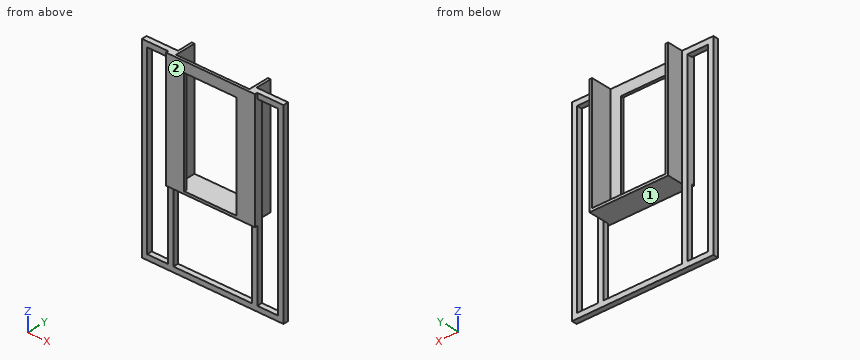
Autodesk Inventor part; units mm, degrees
ref_plane "Work Plane1" through (-336.3192, 12.7, -902.3714) normal (1, 0, 0) x (0, -1, 0)
ref_plane "YZ Plane" through (0, 0, 0) normal (1, 0, 0) x (0, 1, 0)
ref_plane "XZ Plane" through (0, 0, 0) normal (0, 1, 0) x (-1, 0, 0)
sketch "Sketch1" plane through (0, 0, 0) normal (0, 1, 0) x (-1, 0, 0)
  line L0 (-6.5808, 12.0286) -> (-6.5808, -927.7714)
  line L1 (-6.5808, 12.0286) -> (18.8192, 12.0286)
  line L2 (18.8192, 12.0286) -> (18.8192, -902.3714)
  line L3 (18.8192, -902.3714) -> (653.8192, -902.3714)
  line L4 (653.8192, -902.3714) -> (653.8192, 12.0286)
  line L5 (653.8192, 12.0286) -> (679.2192, 12.0286)
  line L6 (679.2192, 12.0286) -> (679.2192, -927.7714)
  line L7 (679.2192, -927.7714) -> (-6.5808, -927.7714)
  line L8 (18.8192, 12.0286) -> (145.8192, 12.0286)
  line L9 (145.8192, 12.0286) -> (145.8192, -902.3714)
  line L10 (145.8192, -902.3714) -> (120.4192, -902.3714)
  line L11 (120.4192, -902.3714) -> (120.4192, 12.0286)
  line L12 (120.4192, -13.8644) -> (18.8192, -13.8644)
  line L13 (653.8192, 12.0286) -> (526.8192, 12.0286)
  line L14 (526.8192, 12.0286) -> (526.8192, -902.3714)
  line L15 (552.2192, 12.0286) -> (552.2192, -902.3714)
  line L16 (552.2192, -13.8644) -> (653.8192, -13.8644)
  point P0 (69.6192, -13.8644)
  dimension "d0" = 939.8
  dimension "d1" = 25.4
  dimension "d2" = 914.4
  dimension "d3" = 635
  dimension "d5" = 25.4
  dimension "d6" = 90
  dimension "d9" = 127
  dimension "d11" = 25.4
  dimension "d12" = 127
  dimension "d21" = 25.4
extrude "Extrusion1" add sketch "Sketch1" along normal mid plane 25.4 contours L1 L2 L3 L4 L5 L6 L7 L0 | L8 L11 L12 L2 | L8 L9 L3 L11 | L4 L16 L15 L13 | L15 L3 L14 L13
sketch "Sketch2" plane through (-526.8192, -12.7, -902.3714) normal (1, 0, 0) x (0, 0, -1)
  line L0 (-914.4, 0) -> (-355.6, 0)
  line L1 (-355.6, 0) -> (-355.6, 101.6)
  line L2 (-355.6, 101.6) -> (-914.4, 101.6)
  line L3 (-914.4, 101.6) -> (-914.4, 0)
  dimension "d14" = 558.8
  dimension "d16" = 101.6
extrude "Extrusion2" add sketch "Sketch2" along normal blind 12.7
ref_plane "Work Plane1" through (-336.3192, 12.7, -902.3714) normal (1, 0, 0) x (0, -1, 0)
mirror "Mirror1" about plane through (-336.3192, 12.7, -902.3714) normal (1, 0, 0) of "Extrusion2"
sketch "Sketch3" plane through (-145.8192, 12.7, -546.7714) normal (0, 0, -1) x (-1, 0, 0)
  line L0 (0, 76.2) -> (381, 76.2)
  line L1 (381, 76.2) -> (381, -25.4)
  line L2 (381, -25.4) -> (0, -25.4)
  line L3 (0, -25.4) -> (0, 76.2)
extrude "Extrusion3" add sketch "Sketch3" along normal blind 12.7
sketch "Sketch4" plane through (0, -12.7, 0) normal (0, -1, 0) x (1, 0, 0)
  line L0 (6.5808, 12.0286) -> (-158.5192, 12.0286)
  line L1 (-552.2192, -902.3714) -> (-552.2192, -13.8644)
  line L2 (-552.2192, -559.4714) -> (-120.4192, -559.4714)
  line L3 (-120.4192, -559.4714) -> (-120.4192, 12.0286)
  line L4 (-120.4192, 12.0286) -> (-552.2192, 12.0286)
  line L5 (-552.2192, 12.0286) -> (-552.2192, -559.4714)
extrude "Extrusion4" add sketch "Sketch4" along normal blind 12.7
sketch "Sketch5" plane through (0, -12.7, 0) normal (0, 1, 0) x (1, 0, 0)
  line L0 (-514.1192, -12.0286) -> (-514.1192, 546.7714)
  line L1 (-158.5192, 546.7714) -> (-514.1192, 546.7714)
  line L2 (-463.3192, 546.7714) -> (-209.3192, 546.7714)
  line L3 (-209.3192, 546.7714) -> (-209.3192, 38.7714)
  line L4 (-209.3192, 38.7714) -> (-463.3192, 38.7714)
  line L5 (-463.3192, 38.7714) -> (-463.3192, 546.7714)
  point P0 (-336.3192, 38.7714)
  dimension "d24" = 254
  dimension "d25" = 508
  dimension "d26" = 177.8
extrude "Extrusion5" cut sketch "Sketch5" against normal blind 12.7
properties part number "Robot frame"
Can you work these out from the model? Positions are in its coordinate system, mm. Face numbers are marked on the shaded views. Coordinates: 2 decimals unless noted, no trailing zeros. Write each loop counter-clockwise with the first axis right and the second up, starting at its lowest first coordinate (ties: lowest second). Pieces come first, ordered by that corner, then holes. Notation, with made-up numbers: (40.5, 57.5) - (81.5, 57.5) arc R29 ccw to (81.5, 83.5) - close; hole circle Ø7 at (62, 66). An arc over 180 degrees is marked (long way). Return JSON: item names as keys, results as strings.
Q1. If we section it at B-B (x = -411.5): Please give me the cut outline in (y, z).
Computed values:
{"outline": "(-25.4, -559.47) - (88.9, -559.47) - (88.9, -546.77) - (-25.4, -546.77) - close; (-25.4, -38.77) - (-12.7, -38.77) - (-12.7, 12.03) - (-25.4, 12.03) - close; (-12.7, -927.77) - (12.7, -927.77) - (12.7, -902.37) - (-12.7, -902.37) - close"}
Q2. If we section it at C-C (x = -586.5): Please give me the cut outline in (y, z).
Computed values:
{"outline": "(-12.7, -927.77) - (12.7, -927.77) - (12.7, -902.37) - (-12.7, -902.37) - close; (-12.7, -13.86) - (12.7, -13.86) - (12.7, 12.03) - (-12.7, 12.03) - close"}
Q3. If we section it at D-D (y = 57.5): Please give me the cut outline in (x, z).
Computed values:
{"outline": "(-526.82, -559.47) - (-145.82, -559.47) - (-145.82, 12.03) - (-158.52, 12.03) - (-158.52, -546.77) - (-514.12, -546.77) - (-514.12, 12.03) - (-526.82, 12.03) - close"}
Q4. Thinking about a two-plate mould opening in Z: for the marked faces 1 and 2, which applies, +Z half, -Z half, draft (parallel to the pull), parting line (faces both ways), or undercut?
Computed values:
{"face 1": "undercut", "face 2": "draft"}
Q5. If we section it at A-A (z = -77): Please give me the cut outline in (x, y).
Computed values:
{"outline": "(-679.22, -12.7) - (-653.82, -12.7) - (-653.82, 12.7) - (-679.22, 12.7) - close; (-552.22, -25.4) - (-463.32, -25.4) - (-463.32, -12.7) - (-514.12, -12.7) - (-514.12, 88.9) - (-526.82, 88.9) - (-526.82, 12.7) - (-552.22, 12.7) - close; (-209.32, -25.4) - (-120.42, -25.4) - (-120.42, 12.7) - (-145.82, 12.7) - (-145.82, 88.9) - (-158.52, 88.9) - (-158.52, -12.7) - (-209.32, -12.7) - close; (-18.82, -12.7) - (6.58, -12.7) - (6.58, 12.7) - (-18.82, 12.7) - close"}
Q6. Please list where these lines run through material, in increasing order: L1, parallel to X at y = -5, z = -263.5; L2, parallel to X at y = -3, z = -688; L3, parallel to X at y = 46, z = -294. Write a range as from..to.
Computed values:
{"L1": "x = -679.22..-653.82, -552.22..-514.12, -158.52..-120.42, -18.82..6.58", "L2": "x = -679.22..-653.82, -552.22..-526.82, -145.82..-120.42, -18.82..6.58", "L3": "x = -526.82..-514.12, -158.52..-145.82"}
Q7. I'm going to push flat-ended pins straight in: pin 1 Ø10 at (y, z) = (39, -424.5) entering from +X; pin 2 Ø1 at (x, y) = (-301, 49) entering from -Z; pin 3 Ø10 at (y, z) = (-19.5, -224) entering from -X. Where does each tip first touch, or does it pass through?
Computed values:
{"pin 1": "stops at x = -145.82", "pin 2": "stops at z = -559.47", "pin 3": "stops at x = -552.22"}
